```python
from build123d import *

# Parameters (mm, degrees)
EXTRUDE_1_DEPTH     = 25
SKETCH_2_R          = 2
CUT_EXTRUDE_1_DEPTH = 41
SKETCH_3_R          = 2.5
CUT_EXTRUDE_2_DEPTH = 10


with BuildPart() as part:
    # 草图1 → 凸台-拉伸1 (new body, symmetric)
    with BuildSketch(Plane(origin=(0, 0, 0), x_dir=(0, 0, -1), z_dir=(1, 0, 0))):
        Polygon((18, 33), (18, 0), (20, 0), (20, 35), (-20, 35), (-20, 0), (-18, 0), (-18, 33), align=None)
    extrude(amount=EXTRUDE_1_DEPTH, both=True)

    # 草图2 → 切除-拉伸1 (cut, through all)
    with BuildSketch(Plane.XY.offset(20)):
        with Locations((-14, 9)):
            Circle(SKETCH_2_R)
        with Locations((14, 9)):
            Circle(SKETCH_2_R)
    extrude(amount=-CUT_EXTRUDE_1_DEPTH, mode=Mode.SUBTRACT)

    # 草图3 → 切除-拉伸2 (cut)
    with BuildSketch(Plane(origin=(0, 35, 0), x_dir=(1, 0, 0), z_dir=(0, 1, 0))):
        with Locations((-20, 0)):
            Circle(SKETCH_3_R)
        with Locations((20, 0)):
            Circle(SKETCH_3_R)
    extrude(amount=-CUT_EXTRUDE_2_DEPTH, mode=Mode.SUBTRACT)


solid = part.part
```
Geometry: final body of the model. Coordinates: model frame, mm. A direction names the side the tool comes from. Round coordinates to 2 decimals unless told otherwise and drop trailing zeros. Loops run counter-clockwise (first coordinate to the right, second up) from the corner with the lowest first, then second, coordinate; pieces in that order, holes last.
Item 1: Line query: L1, parallel to Z at x = -20.5, y = 30; L2, parallel to Y at x = -14, z = 19.25; L3, parallel to Y at x = -2, z = -3. Output: solid intervals per line, ascending.
Checked values:
L1: z = -20 to -18, 18 to 20
L2: y = 0 to 7, 11 to 35
L3: y = 33 to 35
Item 2: Mould query, pull axis Y, two halves, no side actions, for faces 3 (the cylindrical face through (12.526, 10.352, 19.014)), 4 (the flat face through (0, 0, -19)), 5 (the flat face through (0, 16, 18)). Classes: released by +Y, released by -Y, zero draft, split by the parting line, or undercut.
Checked values:
face 3: undercut
face 4: released by -Y
face 5: zero draft
Item 3: Reachability of faces 1 (the flat face through (0, 17, -18)), 2 (the cylindrical face through (-14, 11, -19)) from +Z, -Z, +X, -X, +Y, -Y: full face, straight path, thin tool, end or side. Return the list, or none.
Checked values:
face 1: +X, -X, -Y
face 2: +Z, -Z
Item 4: Section D-D, the plane y = 9. Output: boundary loops of the cut face in (x, z).
Checked values:
outline: (-25, -20) - (-16, -20) - (-16, -18) - (-25, -18) - close; (-25, 18) - (-16, 18) - (-16, 20) - (-25, 20) - close; (-12, -20) - (12, -20) - (12, -18) - (-12, -18) - close; (-12, 18) - (12, 18) - (12, 20) - (-12, 20) - close; (16, -20) - (25, -20) - (25, -18) - (16, -18) - close; (16, 18) - (25, 18) - (25, 20) - (16, 20) - close
Item 5: Section A-A, the plane y = 15. Output: boundary loops of the cut face in (x, z).
Checked values:
outline: (-25, -20) - (25, -20) - (25, -18) - (-25, -18) - close; (-25, 18) - (25, 18) - (25, 20) - (-25, 20) - close
Item 6: Contact query for flat-ended pins moving along their axis: P1, Ø1, axis at x = -3.5, z = -1, coming from the -Y side; P2, Ø6.5, axis at x = -14, y = 9, coming from the -Z side. Output: stop coordinate, or through.
Checked values:
P1: stops at y = 33
P2: stops at z = -20
Item 7: Section C-C, the plane z = 0. Output: boundary loops of the cut face in (x, y).
Checked values:
outline: (-25, 33) - (-22.5, 33) - (-22.5, 35) - (-25, 35) - close; (-17.5, 33) - (17.5, 33) - (17.5, 35) - (-17.5, 35) - close; (22.5, 33) - (25, 33) - (25, 35) - (22.5, 35) - close
Item 8: Section B-B, the plane x = -20. Output: boundary loops of the cut face in (y, z).
Checked values:
outline: (0, -20) - (35, -20) - (35, -2.5) - (33, -2.5) - (33, -18) - (0, -18) - close; (0, 18) - (33, 18) - (33, 2.5) - (35, 2.5) - (35, 20) - (0, 20) - close
